Build history of the part. All positions in model axes, mm. Give positions to 0.01 mm unless a question says otherwise; leave off trailing zeros. Loops run counter-clockwise (first coordinate to the right, second up) from the corner with the lowest first, then second, coordinate; pieces in that order, holes last.
1) Flat gauge pins, fed straight in: P1, Ø5.5, axis at y = -7.94, z = -132.16, coming from the -X side; P2, Ø1, axis at x = 3.5, z = -33.5, coming from the -Y side; P3, Ø6.5, axis at y = -7, z = -72, coming from the +X side. Where does each tip first touch, or does it go through?
2) Wall check: line 1 (X direction, y = -12.5, z = -85.5); line 2 (Y direction, x = 14.5, z = -122); line 3 (Y direction, x = 12.25, z = -159). Give the ranges that are in metal, low to high.
3) Band-saw the part on A-A on z = -222. List the corners of the cut face in (x, y), then the cut area to 3 significant figures.
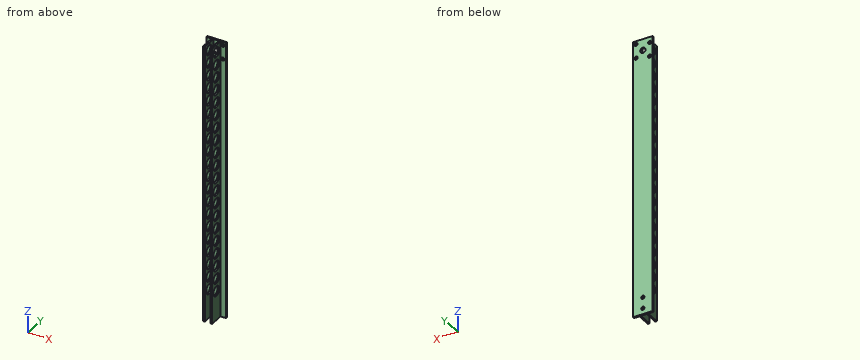
Autodesk Inventor part; units mm, degrees
ref_plane "YZ Plane" through (0, 0, 0) normal (1, 0, 0) x (0, 1, 0)
ref_plane "XZ Plane" through (0, 0, 0) normal (0, 1, 0) x (-1, 0, 0)
ref_plane "XY Plane" through (0, 0, 0) normal (0, 0, 1) x (1, 0, 0)
sketch "Sketch1" plane through (0, 0, 0) normal (0, 0, 1) x (1, 0, 0)
  line L0 (0, 0) -> (17.526, 0)
  line L1 (17.526, 0) -> (17.526, -1.524)
  line L2 (17.526, -1.524) -> (12.7762, -1.524)
  line L3 (12.7762, -1.524) -> (12.7762, -14.351)
  line L4 (12.7762, -14.351) -> (11.2522, -14.351)
  line L5 (11.2522, -14.351) -> (11.2522, -1.524)
  line L6 (11.2522, -1.524) -> (6.2738, -1.524)
  line L7 (6.2738, -1.524) -> (6.2738, -14.351)
  line L8 (6.2738, -14.351) -> (4.7498, -14.351)
  line L9 (4.7498, -14.351) -> (4.7498, -1.524)
  line L10 (4.7498, -1.524) -> (0, -1.524)
  line L11 (0, -1.524) -> (0, 0)
  dimension "d0" = 17.526
  dimension "d1" = 1.524
  dimension "d2" = 4.7498
  dimension "d3" = 12.827
  dimension "d4" = 1.524
  dimension "d5" = 4.9784
  dimension "d6" = 1.524
extrude "Extrusion1" add sketch "Sketch1" against normal blind 249.9995
sketch "Sketch2" plane through (0, 0, 0) normal (0, 1, 0) x (1, 0, 0)
  line L0 (0, 0) -> (17.526, 0)
  line L1 (0, 0) -> (0, 249.9995)
  line L2 (8.763, 0) -> (8.763, 10.16)
  circle A0 centre (8.763, 10.16) radius 2.413
  circle A1 centre (8.763, 10.16) radius 9.5
  circle A2 centre (8.763, 10.16) radius 8
  line L3 (8.763, 10.16) -> (2.6565, 17.4374)
  line L4 (8.763, 10.16) -> (18.263, 10.16) construction
  line L5 (8.763, 10.16) -> (14.8695, 2.8826)
  line L6 (8.763, 10.16) -> (2.6346, 5.0177)
  line L7 (8.763, 10.16) -> (14.8914, 15.3023)
  circle A3 centre (2.6346, 5.0177) radius 1.5
  circle A4 centre (2.6565, 17.4374) radius 1.5
  circle A5 centre (14.8914, 15.3023) radius 1.5
  circle A6 centre (14.8695, 2.8826) radius 1.5
  dimension "d9" = 10.16
  dimension "d10" = 4.826
  dimension "d11" = 19
  dimension "d12" = 16
  dimension "d13" = 130
  dimension "d14" = 3
  dimension "d15" = 3
  dimension "d16" = 3
  dimension "d17" = 3
extrude "Extrusion2" cut sketch "Sketch2" against normal blind 1.524 contours A3 A2 | A6 L5 A1 | A1 A6 | A4 A1 | A1 L3 A4 | A3 L6 A2 | A2 L6 A3 | A0 L6 L2 | L2 L5 A0 | A6 A1 L5 | A1 A4 L3 | L6 A0 L3 | L7 A0 L5 | L3 A0 L7 | A5 A2 | A2 L7 A5 | A5 L7 A2
sketch "Sketch3" plane through (0, 0, 0) normal (0, 1, 0) x (1, 0, 0)
  line L0 (0, 249.9995) -> (17.526, 249.9995)
  line L1 (0, 0) -> (0, 249.9995)
  line L2 (8.763, 249.9995) -> (8.763, 244.6655)
  line L3 (8.763, 244.6655) -> (8.763, 234.6579)
  circle A0 centre (8.763, 244.6655) radius 1.5
  circle A1 centre (8.763, 234.6579) radius 1.5
  dimension "d20" = 5.334
  dimension "d21" = 10.0076
  dimension "d22" = 3
  dimension "d23" = 3
extrude "Extrusion3" cut sketch "Sketch3" against normal blind 1.524
sketch "Sketch5" plane through (12.7762, -14.351, 0) normal (1, 0, 0) x (0, 0, -1)
  line L0 (0, 12.827) -> (0, 0)
  line L1 (0, 0) -> (249.9995, 0)
  line L2 (0, 12.827) -> (249.9995, 12.827)
  line L3 (0, 6.4135) -> (6.4262, 6.4135)
  circle A0 centre (6.4262, 6.4135) radius 4.445
  circle A1 centre (17.8562, 6.4135) radius 4.445
  circle A2 centre (29.2862, 6.4135) radius 4.445
  circle A3 centre (40.7162, 6.4135) radius 4.445
  circle A4 centre (52.1462, 6.4135) radius 4.445
  circle A5 centre (63.5762, 6.4135) radius 4.445
  circle A6 centre (75.0062, 6.4135) radius 4.445
  circle A7 centre (86.4362, 6.4135) radius 4.445
  circle A8 centre (97.8662, 6.4135) radius 4.445
  circle A9 centre (109.2962, 6.4135) radius 4.445
  circle A10 centre (120.7262, 6.4135) radius 4.445
  circle A11 centre (132.1562, 6.4135) radius 4.445
  circle A12 centre (143.5862, 6.4135) radius 4.445
  circle A13 centre (155.0162, 6.4135) radius 4.445
  circle A14 centre (166.4462, 6.4135) radius 4.445
  circle A15 centre (177.8762, 6.4135) radius 4.445
  circle A16 centre (189.3062, 6.4135) radius 4.445
  circle A17 centre (200.7362, 6.4135) radius 4.445
  circle A18 centre (212.1662, 6.4135) radius 4.445
  circle A19 centre (223.5962, 6.4135) radius 4.445
  point P0 (0, 14.351)
  dimension "d38" = 6.4262
  dimension "d39" = 8.89
  dimension "d42" = 11.43
extrude "Extrusion4" cut sketch "Sketch5" against normal blind 25.4
properties part number "Arm_light"
Findings below:
1. P1: passes through
1. P2: stops at y = -1.52
1. P3: stops at x = 12.78
2. line 1: x = 4.75 to 6.27, 11.25 to 12.78
2. line 2: y = -1.52 to 0
2. line 3: y = -14.35 to -9.91, -5.97 to 0
3. outline: (0, -1.52) - (4.75, -1.52) - (4.75, -3.79) - (6.27, -3.79) - (6.27, -1.52) - (11.25, -1.52) - (11.25, -3.79) - (12.78, -3.79) - (12.78, -1.52) - (17.53, -1.52) - (17.53, 0) - (0, 0) - close; (4.75, -14.35) - (6.27, -14.35) - (6.27, -12.09) - (4.75, -12.09) - close; (11.25, -14.35) - (12.78, -14.35) - (12.78, -12.09) - (11.25, -12.09) - close
3. area: 40.5 mm2
